from build123d import *

# Parameters (mm, degrees)
SKIZZE1_W                       = 18
SKIZZE1_H                       = 17
AUFSATZ_LINEAR_AUSTRAGEN1_DEPTH = 2.5
AUFSATZ_LINEAR_AUSTRAGEN2_DEPTH = 3
SKIZZE3_R                       = 1.275
SCHNITT_LINEAR_AUSTRAGEN1_DEPTH = 3.5


with BuildPart() as part:
    # Skizze1 → Aufsatz-Linear austragen1 (new body)
    with BuildSketch(Plane.XY):
        with Locations((9, 8.5)):
            Rectangle(SKIZZE1_W, SKIZZE1_H)
    extrude(amount=AUFSATZ_LINEAR_AUSTRAGEN1_DEPTH)

    # Skizze2 → Aufsatz-Linear austragen2 (add)
    with BuildSketch(Plane.XY.offset(2.5)):
        with BuildLine():
            Line((0.7, 16.4), (0.7, 1.7))
            Line((0.7, 1.7), (13.757142947, 1.7))
            ThreePointArc((13.757142947, 1.7), (14.677664466, 3.922335534), (16.9, 4.842857053))
            Line((16.9, 4.842857053), (16.9, 15))
            Line((16.9, 15), (15.5, 16.4))
            Line((15.5, 16.4), (0.7, 16.4))
        make_face()
    extrude(amount=AUFSATZ_LINEAR_AUSTRAGEN2_DEPTH)

    # Skizze3 → Schnitt-Linear austragen1 (cut, through all)
    with BuildSketch(Plane.XY.offset(2.5)):
        with Locations((16.079023471, 2.15759118)):
            Circle(SKIZZE3_R)
    extrude(amount=-SCHNITT_LINEAR_AUSTRAGEN1_DEPTH, mode=Mode.SUBTRACT)


solid = part.part
Can you work these out from the model? Positions are in its coordinate system, mm. A direction names the side the tool comes from. Coordinates: 2 decimals unless noted, no trailing zeros. Write each loop counter-clockwise with the first axis right and the second up, starting at its lowest first coordinate (ties: lowest second). Pieces come first, ordered by that corner, then holes. Notation, with made-up numbers: (55.25, 6) - (111.25, 6) arc R24 cw to (111.25, 45) - close; hole circle Ø10 at (35.25, -33.75). An arc over 180 degrees is marked (long way). Return JSON: item names as keys, results as strings. Group by question number.
Item 1: I'm going to push flat-ended pins straight in: pin 1 Ø1 at (y, z) = (12.5, 3.5) entering from +X; pin 2 Ø0.9 at (y, z) = (8.5, 4.5) entering from -X; pin 3 Ø1.5 at (x, z) = (13, 3.5) entering from -Y. Where does each tip first touch, or does it pass through?
Item 2: If we section it at B-B (z = 4.7): Write out the boundary of the cut face in (x, y).
Item 3: Which directions (+Z, -Z, +X, -X, +Y, -Y) give clear straight access to the entire face, cutting with the end or side of a thin tool? Please do faces 5 (the face through (16.9, 10, 4)), 6 (the face through (8, 16.4, 4)), 7 (the face through (0.7, 9, 4)), 8 (the face through (7, 1.7, 4)).
Item 4: If we section it at A-A (y = 9.75): Write out the boundary of the cut face in (x, z), then the cut area to 3 significant figures.
Item 5: Please list where these lines run through material, in increasing order: probe 1 along Y at (x, z) = (2.75, 3.2); probe 2 along X at (y, z) = (14.75, 3.55); probe 3 along X at (y, z) = (3.25, 1.5).
Item 6: We'd pull the mould along X, two halves only. Please class faces 1 (the face through (14.805, 2.214, 1.268)), 2 (the face through (16.2, 15.7, 4)), 3 (the face through (0, 8, 1)), 4 (the face through (9, 17, 1)): pulls with the +X half, pulls with the -X half, needs draft (parallel to the pull), parting line crosses it, or undercut.
Item 7: If we section it at C-C (x = 11.25): Write out the boundary of the cut face in (y, z), then the cut area to 3 significant figures.
Return value:
{
 "1": {"pin 1": "stops at x = 16.9", "pin 2": "stops at x = 0.7", "pin 3": "stops at y = 1.7"},
 "2": {"outline": "(0.7, 1.7) - (13.76, 1.7) arc R3.14 cw to (16.9, 4.84) - (16.9, 15) - (15.5, 16.4) - (0.7, 16.4) - close"},
 "3": {"face 5": "+Z, +X, +Y, -Y", "face 6": "+Z, +X, -X, +Y", "face 7": "+Z, -X, +Y, -Y", "face 8": "+Z, +X, -X, -Y"},
 "4": {"outline": "(0, 0) - (18, 0) - (18, 2.5) - (16.9, 2.5) - (16.9, 5.5) - (0.7, 5.5) - (0.7, 2.5) - (0, 2.5) - close", "area": "93.6 mm^2"},
 "5": {"probe 1": "y = 1.7 to 16.4", "probe 2": "x = 0.7 to 16.9", "probe 3": "x = 0 to 15.42, 16.74 to 18"},
 "6": {"face 1": "undercut", "face 2": "pulls with the +X half", "face 3": "pulls with the -X half", "face 4": "needs draft"},
 "7": {"outline": "(0, 0) - (17, 0) - (17, 2.5) - (16.4, 2.5) - (16.4, 5.5) - (1.7, 5.5) - (1.7, 2.5) - (0, 2.5) - close", "area": "86.6 mm^2"}
}
